Could you check a few things on this model? Use its own coordinates, in mm. A direction names the side the tool comes from. Give positions to 0.01 mm unless a question says otherwise; leave off trailing zeros. Loops run counter-clockwise (first coordinate to the right, second up) from the corner with the lowest first, then second, coordinate; pieces in that order, holes last. Notation, with made-up numbers: M 36,37.5 L 47,37.5 A19 ccw 47,49.5 Z; hole C 47,-31.75 d8. An arc over 180 degrees is marked long. Answer in a Markdown table with one row per item. Add a question column.
1. If we section it at A-A on x = 0: List the corners of the cut face in (y, z) for me.
2. If we section it at B-B on z = 0: List the corners of the cut face in (x, y) for me.
3. I need wall thicknesses on line 1 along X through (y, z) = (33, 25); line 2 along X through (y, z) = (-392.5, 1). Which ranges of each line are inside material? Lowest first, please. Write a range as from..to.
4. If we section it at D-D on z = -88.5: List the corners of the cut face in (x, y) for me.
5. I'm going to push flat-ended pins straight in: pin 1 Ø2 at (x, y) = (-83, -288.5) entering from -Z; pin 2 Ø12 at (y, z) = (-226, -100) entering from -X; pin 3 Ø1.5 at (x, y) = (38, -79.5) entering from +Z. Where does each tip first touch, or does it pass through?
6. If we section it at C-C on y = -285: List the corners of the cut face in (x, z) for me, then the cut area to 3 significant figures.
7. Which directions (+Z, -Z, +X, -X, +Y, -Y) give clear straight access to the entire face, cutting with the end or side of a thin tool? Please do faces 1 (the flat face through (-1, 175, 76.2)), 2 (the flat face through (-83, 0, 2)), 3 (the flat face through (76.2, 175, 1)).
```python
from build123d import *

# Parameters (mm, degrees)
SKETCH1_W           = 152.4
SKETCH1_H           = 152.4
BOSS_EXTRUDE1_DEPTH = 355.6
FILLET1_R           = 6.35
SKETCH2_R           = 127
BOSS_EXTRUDE2_DEPTH = 457.2


with BuildPart() as part:
    # Sketch1 → Boss-Extrude1 (new body)
    with BuildSketch(Plane(origin=(0, 0, 0), x_dir=(1, 0, 0), z_dir=(0, 1, 0))):
        Rectangle(SKETCH1_W, SKETCH1_H)
    extrude(amount=BOSS_EXTRUDE1_DEPTH)

    # Fillet1
    fillet1_edges = [part.edges().sort_by_distance(p)[0] for p in [
        (-76.2, 177.8, -76.2),
        (76.2, 177.8, -76.2),
        (76.2, 177.8, 76.2),
        (-76.2, 177.8, 76.2),
    ]]
    fillet(fillet1_edges, radius=FILLET1_R)

    # Sketch2 → Boss-Extrude2 (add)
    with BuildSketch(Plane(origin=(0, 0, 0), x_dir=(-1, 0, 0), z_dir=(0, -1, 0))):
        with Locations(Location((0, 0, 0), (0, 0, 90))):
            Circle(SKETCH2_R)
    extrude(amount=BOSS_EXTRUDE2_DEPTH)


solid = part.part
```
Results:
| question | item | result |
|---|---|---|
| 1 | outline | M -457.2,-127 L 0,-127 L 0,-76.2 L 355.6,-76.2 L 355.6,76.2 L 0,76.2 L 0,127 L -457.2,127 Z |
| 2 | outline | M -127,-457.2 L 127,-457.2 L 127,0 L 76.2,0 L 76.2,355.6 L -76.2,355.6 L -76.2,0 L -127,0 Z |
| 3 | line 1 | -76.2..76.2 |
| 3 | line 2 | -127..127 |
| 4 | outline | M -91.09,-457.2 L 91.09,-457.2 L 91.09,0 L -91.09,0 Z |
| 5 | pin 1 | z = -96.98 |
| 5 | pin 2 | x = -85.4 |
| 5 | pin 3 | z = 121.41 |
| 6 | outline | C 0,0 d254 |
| 6 | area | 50,700 mm2 |
| 7 | face 1 | +Z, +X, -X, +Y |
| 7 | face 2 | +Y |
| 7 | face 3 | +Z, -Z, +X, +Y |
